```python
from build123d import *

# Parameters (mm, degrees)
SKETCH1_R           = 2.1
BOSS_EXTRUDE1_DEPTH = 6


with BuildPart() as part:
    # Sketch1 → Boss-Extrude1 (new body)
    with BuildSketch(Plane.XY):
        with BuildLine():
            ThreePointArc((3.511536297, -3.559369724), (24.301233146, 10.179806707), (48.75, 15))
            ThreePointArc((48.75, 15), (53.723907193, 20.510144327), (47.735035784, 24.895901106))
            ThreePointArc((47.735035784, 24.895901106), (0, 20), (-47.735035784, 24.895901106))
            ThreePointArc((-47.735035784, 24.895901106), (-53.723907193, 20.510144327), (-48.75, 15))
            ThreePointArc((-48.75, 15), (-24.301233146, 10.179806707), (-3.511536297, -3.559369724))
            ThreePointArc((-3.511536297, -3.559369724), (0, -5), (3.511536297, -3.559369724))
        make_face()
        Circle(SKETCH1_R, mode=Mode.SUBTRACT)
        with Locations((-48.75, 20)):
            Circle(SKETCH1_R, mode=Mode.SUBTRACT)
        with Locations((48.75, 20)):
            Circle(SKETCH1_R, mode=Mode.SUBTRACT)
    extrude(amount=BOSS_EXTRUDE1_DEPTH)


solid = part.part
```
The listing builds one solid part. Answer for the finished solid, in the listing's coordinates (mm). Give positions to 0.01 mm unless a question says otherwise; leave off trailing zeros. Order: outer loops, then holes, each group sorted by start corner. A loop starts at its lowest first (then second) coordinate and runs counter-clockwise, first axis right, second up. Notation, with made-up numbers: M 20,60.25 L 77,60.25 A23 ccw 77,81.25 Z; hole C 32.5,-25 d8. An arc over 180 degrees is marked long. Put each result on its own line as item: value. Start each with the question number.
Item 1: Flat-ended cylindrical pins translate along their axes: P1, Ø2, axis at x = 10, z = 3, coming from the -Y side; P2, Ø1.5, axis at y = -1, z = 1, coming from the +X side. Find the tip coordinate at first contact, or state that the pin passes through.
Item 2: The part is cut by section D-D, the plane x = 44. Determine the outline of the cut face in (y, z).
Item 3: The part is cut by section C-C, the plane y = 0. Determine the outline of the cut face in (x, z), and give its area (3 significant figures).
Item 4: The part is cut by section B-B, the plane z = 2.65. Determine the outline of the cut face in (x, y), and give its area (3 significant figures).
Item 5: The part is cut by section A-A, the plane x = 0. Determine the outline of the cut face in (y, z), and give its area (3 significant figures).
Item 6: Find the intervals of material crossed by line 1 along Y through (x, z) = (48, 2.25); line 2 along X through (y, z) = (0.5, 3.1); line 3 along X through (y, z) = (5.5, 1.25), in increasing order.
Item 7: For a pull along X with two mould halves and no side action, classify faces 1 (the face through (49.88, 21.77, 2.96)), 2 (the face through (23.977, 10.046, 2.958)), 3 (the face through (0, -5, 3)) as +X half, -X half, draft (parallel to the pull), parting line (faces both ways), or undercut.
Answer key:
1. P1: stops at y = 1.27
1. P2: stops at x = 7.13
2. outline: M 14.82,0 L 24.15,0 L 24.15,6 L 14.82,6 Z
3. outline: M -7.43,0 L -2.1,0 L -2.1,6 L -7.43,6 Z; M 2.1,0 L 7.43,0 L 7.43,6 L 2.1,6 Z
3. area: 63.9 mm²
4. outline: M -48.75,15 A64.41 cw -3.51,-3.56 A5 ccw 3.51,-3.56 A64.41 cw 48.75,15 A5 ccw long 47.74,24.9 A235.16 cw -47.74,24.9 A5 ccw long Z; hole C -48.75,20 d4.2; hole C 0,0 d4.2; hole C 48.75,20 d4.2
4. area: 1,350 mm²
5. outline: M -5,0 L -2.1,0 L -2.1,6 L -5,6 Z; M 2.1,0 L 20,0 L 20,6 L 2.1,6 Z
5. area: 125 mm²
6. line 1: y = 15 to 18.04, 21.96 to 24.94
6. line 2: x = -8.03 to -2.04, 2.04 to 8.03
6. line 3: x = -15.08 to 15.08
7. face 1: undercut
7. face 2: +X half
7. face 3: parting line
